Verification items for the finished model (mm, model axes). Round coordinates to 2 decimals unless told otherwise and drop trailing zeros. Write each loop counter-clockwise with the first axis right and the second up, starting at its lowest first coordinate (ties: lowest second). Pieces come first, ordered by that corner, then holes. Notation, with made-up numbers: M 0.25,80.5 L 50.25,80.5 A26 ccw 50.25,119.5 Z; hole C 49.5,20 d4. An arc over 180 degrees is marked long. One line per question, with ' | ' between items. Start each with the question number.
Q1. Release check for a two-part mould opening along X. For faces 1 (the face through (-25.513, 2.465, -5.195)), 2 (the face through (-30.215, 0.301, -5.056)), 3 (the face through (-15.05, 4.699, -0.285)) record: released by +X, released by -X, zero draft, split by the parting line, or undercut.
Q2. Cross-section at A-A (z = -5). Record the boundary of the cut face in (x, y), then the cut area to 3 significant figures.
Q3. Thickness scan on line 1 along X through (y, z) = (3.7, -5); line 2 along Z through (x, y) = (-27, 1.95); line 3 along X through (y, z) = (4.75, -5). Record the ranges inside material, lowest first. Write a range as from..to.
Q4. Cross-section at D-D (x = -11.5). Record the boundary of the cut face in (y, z).
Q5. Cross-section at C-C (y = 2.5). Record the boundary of the cut face in (x, z), then the cut area to 3 significant figures.
Q6. Cross-section at B-B (x = -3.5). Record the boundary of the cut face in (y, z), then the cut area to 3 significant figures.
from build123d import *

# Parameters (mm, degrees)
SKETCH1_W               = 30.5
SKETCH1_H               = 10
BOSS_EXTRUDE1_DEPTH     = 5
CUT_EXTRUDE1_DEPTH      = 33.484611742
CUT_EXTRUDE1_DEPTH_BACK = 33.484611742
SKETCH2_R               = 1.5
FILLET1_R               = 1


with BuildPart() as part:
    # Sketch1 → Boss-Extrude1 (new body)
    with BuildSketch(Plane(origin=(0, 0, 0), x_dir=(1, 0, 0), z_dir=(0, 1, 0))):
        with Locations((-15.25, 5)):
            Rectangle(SKETCH1_W, SKETCH1_H)
    extrude(amount=BOSS_EXTRUDE1_DEPTH)

    # Sketch2 → Cut-Extrude1 (cut, two sides: drawn at the far end of the back side and taken through both)
    with BuildSketch(Plane(origin=(0, 5, 0), x_dir=(1, 0, 0), z_dir=(0, 1, 0)).offset(-CUT_EXTRUDE1_DEPTH_BACK)):
        with Locations(Location((-27, 5, 0), (0, 0, 270))):
            Circle(SKETCH2_R)
        with Locations(Location((-3.5, 5, 0), (0, 0, 270))):
            Circle(SKETCH2_R)
    extrude(amount=CUT_EXTRUDE1_DEPTH + CUT_EXTRUDE1_DEPTH_BACK, mode=Mode.SUBTRACT)

    # Fillet1
    fillet1_edges = [part.edges().sort_by_distance(p)[0] for p in [
        (-30.5, 5, -5),
        (-15.25, 5, 0),
        (0, 5, -5),
        (-15.25, 0, 0),
        (-30.5, 0, -5),
        (-15.25, 0, -10),
        (0, 0, -5),
        (0, 2.5, 0),
        (-30.5, 2.5, 0),
        (-30.5, 2.5, -10),
        (0, 2.5, -10),
        (-15.25, 5, -10),
    ]]
    fillet(fillet1_edges, radius=FILLET1_R)


solid = part.part
Determined:
1) face 1: undercut | face 2: released by -X | face 3: zero draft
2) outline: M -30.5,1 A1 ccw -29.5,0 L -28.5,0 L -28.5,5 L -29.5,5 A1 ccw -30.5,4 Z; M -25.5,0 L -5,0 L -5,5 L -25.5,5 Z; M -2,0 L -1,0 A1 ccw 0,1 L 0,4 A1 ccw -1,5 L -2,5 Z | area: 122 mm²
3) line 1: x = -30.5..-28.5, -25.5..-5, -2..0 | line 2: z = -10..-6.5, -3.5..0 | line 3: x = -30.16..-28.5, -25.5..-5, -2..-0.34
4) outline: M 0,-9 A1 ccw 1,-10 L 4,-10 A1 ccw 5,-9 L 5,-1 A1 ccw 4,0 L 1,0 A1 ccw 0,-1 Z
5) outline: M -30.5,-9 A1 ccw -29.5,-10 L -1,-10 A1 ccw 0,-9 L 0,-1 A1 ccw -1,0 L -29.5,0 A1 ccw -30.5,-1 Z; hole C -27,-5 d3; hole C -3.5,-5 d3 | area: 290 mm²
6) outline: M 0,-9 A1 ccw 1,-10 L 4,-10 A1 ccw 5,-9 L 5,-6.5 L 0,-6.5 Z; M 0,-3.5 L 5,-3.5 L 5,-1 A1 ccw 4,0 L 1,0 A1 ccw 0,-1 Z | area: 34.1 mm²
